For this review, take the finished solid that the model builds, in its own axes (mm). A direction names the side the tool comes from. Round coordinates to 2 decimals unless told otherwise and drop trailing zeros. Order: outer loops, then holes, each group sorted by start corner. A loop starts at its lowest first (then second) coordinate and runs counter-clockwise, first axis right, second up. Notation, with made-up numbers: (14.25, 14.25) -> (59.25, 14.25) arc R32 ccw to (59.25, 46.25) -> close; hole circle Ø4 at (-22, 50). An arc over 180 degrees is marked (long way). Use a Markdown table: item, result. Add a question column.
1) Consider section D-D (y = -0.5). State the section outline as (x, z) points, plus the area to 3 significant figures.
2) Consider section B-B (y = 1). State the section outline as (x, z) points.
3) Machinability: for faces 1 (the face through (-4, 1, -1.1)), 2 (the face through (-5, 1, 0.3)), 3 (the face through (1.09, 1.16, -0.14)), which of the approach directions +Z, -Z, +X, -X, +Y, -Y give a long, thin tool a straight path to every point of the face, cutting with its end or side? Answer none if there is none.
4) Clearance check with flat-ended pins moving along their axes: P1, Ø1.1, axis at x = -4.5, y = 1, coming from the -Z side; P2, Ø1.1, axis at x = -5.5, y = 0.5, coming from the +Z side; P3, Ø1, axis at y = 0, z = -2, coming from the -X side. State where each tip first meets the part, or that it passes through.
5) Draft analysis for pull direction Z (two halves, no side actions). For faces 4 (the face through (-2.579, 1.085, 0.448)), 5 (the face through (-3, 0, 0)), 6 (the face through (1.31, 1.08, -1.56)), 7 (the face through (-1.1, 1.08, -1.79)), state which applies: pulls with the +Z half, pulls with the -Z half, needs draft (parallel to the pull), parting line crosses it, or undercut.
6) Wall thickness on line 1 along Y through (x, z) = (-1.5, 1.25); line 2 along X through (y, z) = (1.75, -1.6); line 3 along X through (y, z) = (2, -0.45): over which ranges is each line inside the solid? List them lowest first. Write a range as [from, to].
7) Consider section C-C (x = -5.25). State the section outline as (y, z) points.
8) Consider section A-A (z = 0). State the section outline as (x, y) points.
```python
from build123d import *

# Parameters (mm, degrees)
BOSS_EXTRUDE1_DEPTH      = 2.2
BOSS_EXTRUDE2_DEPTH      = 4.4
BOSS_EXTRUDE2_DEPTH_BACK = 2
SKETCH1_3_R              = 1.1
FILLET1_R                = 0.2


with BuildPart() as part:
    # Sketch1 → Boss-Extrude1 (new body)
    with BuildSketch(Plane(origin=(0, 0, 0), x_dir=(1, 0, 0), z_dir=(0, 1, 0))):
        with BuildLine():
            Line((-1.788854382, 1.1), (-7.288854382, 1.1))
            Line((-7.288854382, 1.1), (-7.288854382, -0.3))
            Line((-7.288854382, -0.3), (-3.130458393, -0.3))
            Line((-3.130458393, -0.3), (-2.012601597, -0.599528826))
            ThreePointArc((-2.012601597, -0.599528826), (-1.860410686, -0.974100652), (-1.639259655, -1.312565344))
            Line((-1.639259655, -1.312565344), (-2.048076211, -2.452627944))
            Line((-2.048076211, -2.452627944), (0.55, -0.952627944))
            ThreePointArc((0.55, -0.952627944), (1.095814168, -0.095871317), (0.707066371, 0.842648887))
            Line((0.707066371, 0.842648887), (1.928362829, 2.298133329))
            Line((1.928362829, 2.298133329), (-0.203939042, 2.09007389))
            ThreePointArc((-0.203939042, 2.09007389), (-1.112595158, 1.78104801), (-1.788854382, 1.1))
        make_face()
    extrude(amount=BOSS_EXTRUDE1_DEPTH)

    # Sketch1_3 → Boss-Extrude2 (add, two sides: drawn at the far end of the back side and taken through both)
    with BuildSketch(Plane(origin=(0, 0, 0), x_dir=(1, 0, 0), z_dir=(0, 1, 0)).offset(-BOSS_EXTRUDE2_DEPTH_BACK)):
        with Locations(Location((0, 0, 0), (0, 0, 270))):
            Circle(SKETCH1_3_R)
    extrude(amount=BOSS_EXTRUDE2_DEPTH + BOSS_EXTRUDE2_DEPTH_BACK)

    # Fillet1
    fillet1_edges = [part.edges().sort_by_distance(p)[0] for p in [
        (-7.288854382, 1.1, 0.3),
        (-7.288854382, 1.1, -1.1),
        (-2.048076211, 1.1, 2.452627944),
    ]]
    fillet(fillet1_edges, radius=FILLET1_R)


solid = part.part
```
Results list:
| question | item | result |
|---|---|---|
| 1 | outline | circle Ø2.2 at (0, 0) |
| 1 | area | 3.80 mm2 |
| 2 | outline | (-7.29, -0.9) arc R0.2 ccw to (-7.09, -1.1) -> (-1.79, -1.1) arc R2.1 ccw to (-0.2, -2.09) -> (1.93, -2.3) -> (0.71, -0.84) arc R1.1 ccw to (0.55, 0.95) -> (-1.58, 2.18) arc R0.2 ccw to (-1.86, 1.94) -> (-1.64, 1.31) arc R2.1 ccw to (-2.01, 0.6) -> (-3.13, 0.3) -> (-7.09, 0.3) arc R0.2 ccw to (-7.29, 0.1) -> close |
| 3 | face 1 | -Z, -X, +Y, -Y |
| 3 | face 2 | +Z, -X, +Y, -Y |
| 3 | face 3 | none |
| 4 | P1 | z = -1.1 |
| 4 | P2 | z = 0.3 |
| 4 | P3 | x = -1.47 |
| 5 | face 4 | pulls with the +Z half |
| 5 | face 5 | needs draft |
| 5 | face 6 | undercut |
| 5 | face 7 | pulls with the -Z half |
| 6 | line 1 | [0, 2.2] |
| 6 | line 2 | [-1.36, 1.34] |
| 6 | line 3 | [-7.29, 1] |
| 7 | outline | (0, -1.1) -> (2.2, -1.1) -> (2.2, 0.3) -> (0, 0.3) -> close |
| 8 | outline | (-7.29, 0) -> (-1.1, 0) -> (-1.1, -2) -> (1.1, -2) -> (1.1, 4.4) -> (-1.1, 4.4) -> (-1.1, 2.2) -> (-7.29, 2.2) -> close |
